Autodesk Fusion 360 part; units mm, degrees
sketch "Sketch1" plane through (0, 0, 0) normal (0, 0, 1) x (1, 0, 0)
  line L0 (0, 0) -> (15, 0)
  line L1 (15, 0) -> (15, 15)
  line L2 (15, 15) -> (0, 15)
  line L3 (0, 15) -> (0, 0)
  line L4 (5.1406, 12.0446) -> (9.9406, 12.0446)
  line L5 (9.9406, 12.0446) -> (9.9406, 3.0446)
  line L6 (9.9406, 3.0446) -> (5.1406, 3.0446)
  line L7 (5.1406, 3.0446) -> (5.1406, 12.0446)
  dimension "d1" = 15
  dimension "d2" = 15
  dimension "d3" = 4.8
  dimension "d4" = 9
extrude "Extrude1" add sketch "Sketch1" along normal blind 37.25
sketch "Sketch4" plane through (0, 0, 0) normal (0, 0, 1) x (1, 0, 0)
  line L0 (5.0344, 1.7938) -> (15.0344, 1.7938)
  line L1 (15.0344, 1.7938) -> (15.0344, 13.2938)
  line L2 (15.0344, 13.2938) -> (5.0344, 13.2938)
  line L3 (5.0344, 13.2938) -> (5.0344, 1.7938)
  dimension "d14" = 10
  dimension "d15" = 11.5
extrude "Extrude5" cut sketch "Sketch4" along normal blind 31.25
sketch "Sketch5" plane through (15, 0, 0) normal (1, 0, 0) x (0, 1, 0)
  line L0 (13.2938, 0) -> (15, 0)
  line L1 (15, 0) -> (15, 37.25)
  line L2 (15, 37.25) -> (0, 37.25)
  line L3 (0, 37.25) -> (0, 0)
  line L4 (2.5112, 0) -> (12.5112, 0)
  line L5 (12.5112, 0) -> (12.5112, 25)
  line L6 (12.5112, 25) -> (2.5112, 25)
  line L7 (2.5112, 25) -> (2.5112, 0)
  line L8 (13.2938, 31.25) -> (13.2938, 0)
  line L9 (0, 0) -> (1.7938, 0)
  line L10 (1.7938, 0) -> (1.7938, 31.25)
  line L11 (1.7938, 31.25) -> (13.2938, 31.25)
  dimension "d18" = 25
  dimension "d21" = 10
extrude "Extrude6" cut sketch "Sketch5" against normal blind 7 contours L4 L5 L6 L7
Source: CAD feature listing. Evaluate the final solid. Frame: model axes, mm. A direction names the side the tool comes from. Round coordinates to 2 decimals unless told otherwise and drop trailing zeros. Loops run counter-clockwise (first coordinate to the right, second up) from the corner with the lowest first, then second, coordinate; pieces in that order, holes last. Notation, with made-up numbers: M 13,68 L 31,68 A23 ccw 31,99 Z; hole C -1.5,48.25 d10. An arc over 180 degrees is marked long. Use a Markdown table: item, result. Add a question column.
1. Contact query for flat-ended pins moving along their axis: P1, Ø4, axis at y = 11, z = 28, coming from the +X side; P2, Ø5, axis at x = 7.5, z = 16, coming from the -Y side; P3, Ø1.5, axis at x = 12, y = 11, coming from the -Z side. Output: stop coordinate, or through.
2. Line query: line 1 (Y direction, x = 9, z = 16.5); line 2 (Y direction, x = 5.25, z = 34); line 3 (X direction, y = 5, z = 6). Output: solid intervals per line, ascending.
3. Reachability of faces 1 (the flat face through (10, 13.294, 15)), 2 (the flat face through (9.941, 8, 34)), 3 (the flat face through (0, 8, 18)) from +Z, -Z, +X, -X, +Y, -Y: full face, straight path, thin tool, end or side. Return the list, or none.
4. Section query C-C on z = 27.5. Return the cut outline in (x, y).
5. Section query B-B on y = 10.75. Return the cut outline in (x, z).
6. Section query D-D on y = 12.5. Return the cut outline in (x, z).
7. Mould query, pull axis Y, two halves, no side actions, for faces 4 (the flat face through (8, 15, 18)), 5 (the flat face through (10, 1.794, 15)), 6 (the flat face through (5.034, 8, 15)), 7 (the flat face through (4, 8, 37.25)). Classes: pulls with the +Y half, pulls with the -Y half, needs draft (parallel to the pull), parting line crosses it, or undercut.
8. Section query A-A on x = 6.75. Return the cut outline in (y, z).
Reported:
| question | item | result |
|---|---|---|
| 1 | P1 | stops at x = 5.03 |
| 1 | P2 | stops at y = 0 |
| 1 | P3 | stops at z = 31.25 |
| 2 | line 1 | y = 0 to 1.79, 13.29 to 15 |
| 2 | line 2 | y = 0 to 3.04, 12.04 to 15 |
| 2 | line 3 | x = 0 to 5.03 |
| 3 | face 1 | -Z, +X |
| 3 | face 2 | +Z, -Z |
| 3 | face 3 | +Z, -Z, -X, +Y, -Y |
| 4 | outline | M 0,0 L 15,0 L 15,1.79 L 5.03,1.79 L 5.03,13.29 L 15,13.29 L 15,15 L 0,15 Z |
| 5 | outline | M 0,0 L 5.03,0 L 5.03,31.25 L 5.14,31.25 L 5.14,37.25 L 0,37.25 Z; M 9.94,31.25 L 15,31.25 L 15,37.25 L 9.94,37.25 Z |
| 6 | outline | M 0,0 L 5.03,0 L 5.03,31.25 L 15,31.25 L 15,37.25 L 0,37.25 Z |
| 7 | face 4 | pulls with the +Y half |
| 7 | face 5 | undercut |
| 7 | face 6 | undercut |
| 7 | face 7 | needs draft |
| 8 | outline | M 0,0 L 1.79,0 L 1.79,31.25 L 3.04,31.25 L 3.04,37.25 L 0,37.25 Z; M 12.04,31.25 L 13.29,31.25 L 13.29,0 L 15,0 L 15,37.25 L 12.04,37.25 Z |
